For this review, use the dimensioned drawing (mm, ordinates from the lowest corner) and the shaded views. A direction names the side the tool comes from. Round coordinates to 2 decimals unless told otherwise and drop trailing zeros. Write each loop counter-clockwise with the first axis right and the second up, starting at its lowest first coordinate (ties: lowest second). Pieces come first, ordered by that corner, then holes. Notation, with made-up numbers: M -32.5,80.5 L -27.5,80.5 A10 ccw -27.5,84.5 Z; hole C -16,59 d1. An arc over 180 degrees is marked long. One line per question, with ' | ' between items.
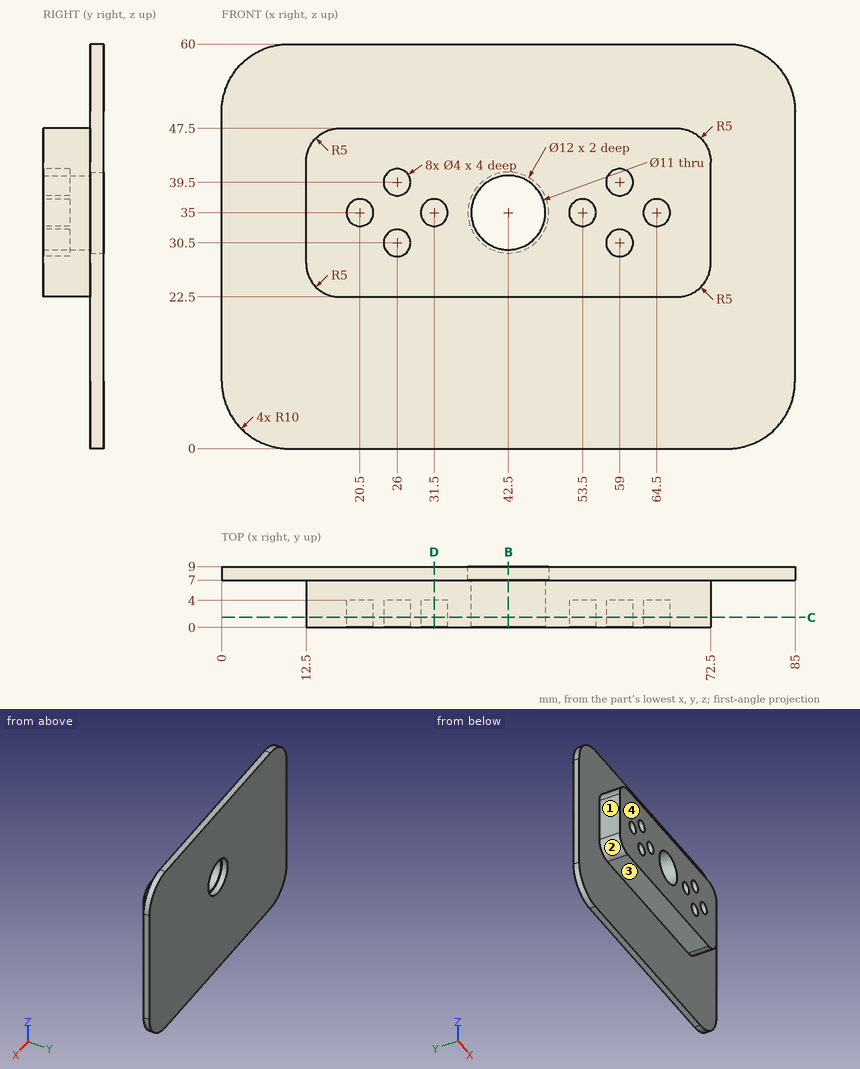
Item 1: Take a section at B-B (x = 42.5). Write out the cut boundary in (y, z).
Results:
outline: M 0,22.5 L 7,22.5 L 7,0 L 9,0 L 9,29 L 7,29 L 7,29.5 L 0,29.5 Z; M 0,40.5 L 7,40.5 L 7,41 L 9,41 L 9,60 L 7,60 L 7,47.5 L 0,47.5 Z
Item 2: Take a section at D-D (x = 31.5). Write out the cut boundary in (y, z).
Results:
outline: M 0,22.5 L 7,22.5 L 7,0 L 9,0 L 9,60 L 7,60 L 7,47.5 L 0,47.5 L 0,37 L 4,37 L 4,33 L 0,33 Z
Item 3: To check wall thickness, follow line 1 along Z through (x, y) = (26, 1.7); line 2 along Z through (x, y) = (20.5, 2.1); line 3 along X through (y, z) = (1, 42). State the ranges of each line that lie inside material, in increasing order. Write a range as from..to.
Results:
line 1: 22.5..28.5, 32.5..37.5, 41.5..47.5 | line 2: 22.5..33, 37..47.5 | line 3: 12.5..72.5
Item 4: Insertion check: pin 1 Ø3.5 at (x, y) = (54, 4) entering from -Z; pin 2 Ø6 at (x, z) = (48.5, 19) entering from -Y; pin 3 Ø4 at (y, z) = (3, 33.5) entering from +X. Each pin has a flat end and moves straight along its axis. Give the tip position at first contact, or say it passes through.
Results:
pin 1: z = 22.5 | pin 2: y = 7 | pin 3: x = 72.5
Item 5: Take a section at C-C (y = 1.5). State how many separate pieces and enclosed holes the cut face has, then the cut area to 3 significant figures.
Results:
separate pieces: 1 | enclosed holes: 9 | area: 1,280 mm2
Item 6: Machinability: for the marked faces 1, 2, 3 and 4, which of the approach directions +Z, -Z, +X, -X, +Y, -Y give a long, thin tool a straight path to every point of the face, cutting with its end or side? Answer none if there is none.
Results:
face 1: +Z, -Z, -X, -Y | face 2: -Z, -X, -Y | face 3: -Z, +X, -X, -Y | face 4: +Z, -Z, +X, -X, -Y
